```python
from build123d import *

# Parameters (mm, degrees)
SKETCH_1_W               = 120
SKETCH_1_H               = 60
EXTRUDE_1_DEPTH          = 5
CUT_EXTRUDE_1_REACH      = 69.268
SKETCH_2_W               = 5
SKETCH_2_H               = 10
PATTERN_LINEAR_1_COUNT   = 3
PATTERN_LINEAR_1_PITCH   = 20
MIRROR_1_COPY_1_REACH    = 69.268
MIRROR_1_COPY_1_SKETCH_W = 5
MIRROR_1_COPY_1_SKETCH_H = 10
MIRROR_1_COPY_2_REACH    = 69.268
MIRROR_1_COPY_2_SKETCH_W = 5
MIRROR_1_COPY_2_SKETCH_H = 10
CUT_EXTRUDE_2_REACH      = 69.268
SKETCH_3_W               = 10
SKETCH_3_H               = 5
PATTERN_LINEAR_2_COUNT   = 3
PATTERN_LINEAR_2_PITCH   = 20
PATTERN_LINEAR_3_COUNT   = 3
PATTERN_LINEAR_3_PITCH   = 20


with BuildPart() as part:
    # 스케치1 → 보스-돌출1 (new body)
    with BuildSketch(Plane.XY):
        Rectangle(SKETCH_1_W, SKETCH_1_H)
    extrude(amount=EXTRUDE_1_DEPTH)

    # 스케치2 → 컷-돌출1 (cut, up to next)
    with BuildSketch(Plane.XY.offset(5), mode=Mode.PRIVATE) as cut_extrude_1_sk1:
        with Locations((-57.5, 25)):
            Rectangle(SKETCH_2_W, SKETCH_2_H)
    cut_extrude_1_tool1 = extrude(cut_extrude_1_sk1.sketch, amount=-CUT_EXTRUDE_1_REACH, mode=Mode.PRIVATE) & part.part
    cut_extrude_1 = cut_extrude_1_tool1.solids().sort_by_distance((-57.5, 25, 5))[0]
    add(cut_extrude_1, mode=Mode.SUBTRACT)

    # 선형 패턴1: 컷-돌출1 ×3
    with Locations(*[(0, -i * PATTERN_LINEAR_1_PITCH, 0) for i in range(1, PATTERN_LINEAR_1_COUNT)]):
        add(cut_extrude_1, mode=Mode.SUBTRACT)

    # 대칭 복사1: 컷-돌출1 across plane
    add(cut_extrude_1.mirror(Plane(origin=(0, 0, 0), x_dir=(0, 0, 1), z_dir=(1, 0, 0))), mode=Mode.SUBTRACT)

    # 대칭 복사1 copy 1 sketch → 대칭 복사1 copy 1 (cut, up to next)
    with BuildSketch(Plane(origin=(0, -20, 5), x_dir=(-1, 0, 0), z_dir=(0, 0, 1)), mode=Mode.PRIVATE) as mirror_1_copy_1_sk1:
        with Locations((-57.5, -25)):
            Rectangle(MIRROR_1_COPY_1_SKETCH_W, MIRROR_1_COPY_1_SKETCH_H)
    mirror_1_copy_1_tool1 = extrude(mirror_1_copy_1_sk1.sketch, amount=-MIRROR_1_COPY_1_REACH, mode=Mode.PRIVATE) & part.part
    add(mirror_1_copy_1_tool1.solids().sort_by_distance((57.5, 5, 5))[0], mode=Mode.SUBTRACT)

    # 대칭 복사1 copy 2 sketch → 대칭 복사1 copy 2 (cut, up to next)
    with BuildSketch(Plane(origin=(0, -40, 5), x_dir=(-1, 0, 0), z_dir=(0, 0, 1)), mode=Mode.PRIVATE) as mirror_1_copy_2_sk1:
        with Locations((-57.5, -25)):
            Rectangle(MIRROR_1_COPY_2_SKETCH_W, MIRROR_1_COPY_2_SKETCH_H)
    mirror_1_copy_2_tool1 = extrude(mirror_1_copy_2_sk1.sketch, amount=-MIRROR_1_COPY_2_REACH, mode=Mode.PRIVATE) & part.part
    add(mirror_1_copy_2_tool1.solids().sort_by_distance((57.5, -15, 5))[0], mode=Mode.SUBTRACT)

    # 스케치3 → 컷-돌출2 (cut, up to next)
    with BuildSketch(Plane.XY.offset(5), mode=Mode.PRIVATE) as cut_extrude_2_sk1:
        with Locations((0, 27.5)):
            Rectangle(SKETCH_3_W, SKETCH_3_H)
    cut_extrude_2_tool1 = extrude(cut_extrude_2_sk1.sketch, amount=-CUT_EXTRUDE_2_REACH, mode=Mode.PRIVATE) & part.part
    cut_extrude_2 = cut_extrude_2_tool1.solids().sort_by_distance((0, 27.5, 5))[0]
    add(cut_extrude_2, mode=Mode.SUBTRACT)

    # 선형 패턴2: 컷-돌출2 ×3
    with Locations(*[(-i * PATTERN_LINEAR_2_PITCH, 0, 0) for i in range(1, PATTERN_LINEAR_2_COUNT)]):
        add(cut_extrude_2, mode=Mode.SUBTRACT)

    # 선형 패턴3: 컷-돌출2 ×3
    with Locations(*[(i * PATTERN_LINEAR_3_PITCH, 0, 0) for i in range(1, PATTERN_LINEAR_3_COUNT)]):
        add(cut_extrude_2, mode=Mode.SUBTRACT)


solid = part.part
```
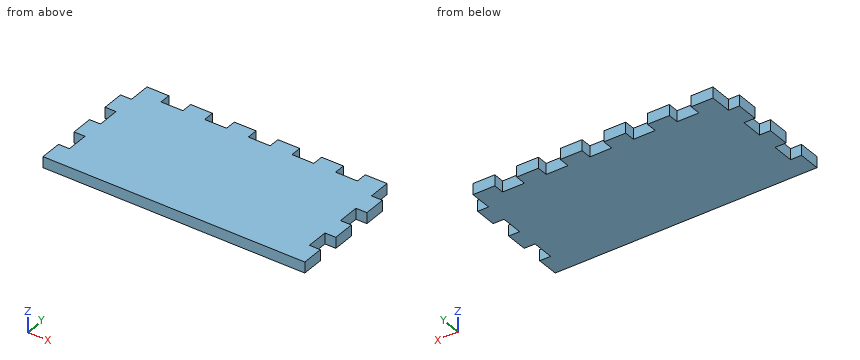
Source: CAD feature listing. Evaluate the final solid. Frame: model axes, mm. Coordinates: 2 decimals unless noted, no trailing zeros. Order: outer loops, then holes, each group sorted by start corner. A loop starts at its lowest first (then second) coordinate and runs counter-clockwise, first axis right, second up. Notation, with made-up numbers: (-5.5, -2) - (40.5, -2) arc R23 ccw to (40.5, 21) - close; hole circle Ø1 at (-7.5, 74). An arc over 180 degrees is marked (long way). One line per item, written item: value.
1) Cut plane B-B on x = -19.5. Output: boundary loops of the cut face in (y, z), plus the area to 3 significant figures.
Computed values:
outline: (-30, 0) - (25, 0) - (25, 5) - (-30, 5) - close
area: 275 mm^2
2) Ray query, line 1 (X direction, y = 25.5, z = 1.6); line 2 (Y direction, x = -43, z = 3.4); line 3 (X direction, y = 8.5, z = 3.95). Return the intervals inside material, ascending. Write a range as [from, to].
Computed values:
line 1: x = [-55, -45], [-35, -25], [-15, -5], [5, 15], [25, 35], [45, 55]
line 2: y = [-30, 25]
line 3: x = [-55, 55]
3) Contact query for flat-ended pins moving along their axis: pin 1 (1.5 mm diameter, centred on x = -0.5, z = 1.5, fed in from +Y); pin 2 (2.5 mm diameter, centred on y = -16, z = 2, fed in from -X). Output: stop coordinate, or through.
Computed values:
pin 1: stops at y = 25
pin 2: stops at x = -55
4) Cut plane A-A on y = 5.5. Output: boundary loops of the cut face in (x, z).
Computed values:
outline: (-55, 0) - (55, 0) - (55, 5) - (-55, 5) - close
